```python
from build123d import *

# Parameters (mm, degrees)
BOSS_EXTRUDE1_DEPTH = 13.25
BOSS_EXTRUDE2_START = -2
BOSS_EXTRUDE2_DEPTH = 2
CHAMFER2_SIZE       = 2.5


with BuildPart() as part:
    # Sketch2 → Boss-Extrude1 (new, symmetric)
    with BuildSketch(Plane(origin=(0, 0, 0), x_dir=(1, 0, 0), z_dir=(0, 1, 0))):
        with BuildLine():
            Line((-52.61897195, 127.03343572), (-52.795575656, 127.459794782))
            Line((-52.795575656, 127.459794782), (-50.947816591, 128.225161647))
            Line((-50.947816591, 128.225161647), (-51.55131776, 129.682142355))
            Line((-51.55131776, 129.682142355), (-53.399076825, 128.91677549))
            Line((-53.399076825, 128.91677549), (-53.575680531, 129.343134552))
            ThreePointArc((-53.575680531, 129.343134552), (0, 140), (53.575680531, 129.343134552))
            Line((53.575680531, 129.343134552), (53.399076825, 128.91677549))
            Line((53.399076825, 128.91677549), (53.360808482, 128.824387537))
            Line((53.360808482, 128.824387537), (55.116179594, 128.097289015))
            Line((55.116179594, 128.097289015), (54.589215111, 126.825084214))
            Line((54.589215111, 126.825084214), (52.833843999, 127.552182735))
            Line((52.833843999, 127.552182735), (52.795575656, 127.459794782))
            Line((52.795575656, 127.459794782), (52.61897195, 127.03343572))
            ThreePointArc((52.61897195, 127.03343572), (0, 137.5), (-52.61897195, 127.03343572))
        make_face()
    extrude(amount=BOSS_EXTRUDE1_DEPTH, both=True)

    # Sketch3 → Boss-Extrude2 (add)
    with BuildSketch(Plane.XZ.offset(13.25).offset(BOSS_EXTRUDE2_START)):
        with BuildLine():
            ThreePointArc((53.575680531, -129.343134552), (0, -140), (-53.575680531, -129.343134552))
            Line((-53.575680531, -129.343134552), (-54.532389112, -131.652833383))
            ThreePointArc((-54.532389112, -131.652833383), (0, -142.5), (54.532389112, -131.652833383))
            Line((54.532389112, -131.652833383), (53.575680531, -129.343134552))
        make_face()
        with BuildLine():
            Line((-51.662263369, -124.723736889), (-52.61897195, -127.03343572))
            ThreePointArc((-52.61897195, -127.03343572), (0, -137.5), (52.61897195, -127.03343572))
            Line((52.61897195, -127.03343572), (51.662263369, -124.723736889))
            ThreePointArc((51.662263369, -124.723736889), (0, -135), (-51.662263369, -124.723736889))
        make_face()
    extrude(amount=BOSS_EXTRUDE2_DEPTH)

    # Chamfer2
    chamfer2_edges = [part.edges().sort_by_distance(p)[0] for p in [
        (0, -11.25, -137.5),
        (0, -11.25, -140),
    ]]
    chamfer(chamfer2_edges, length=CHAMFER2_SIZE - 0.0001)  # a hair under: the kernel refuses the full size


solid = part.part
```
Geometry: final body of the model. Coordinates: model frame, mm. A direction names the side the tool comes from. Round coordinates to 2 decimals unless told otherwise and drop trailing zeros. Write each loop counter-clockwise with the first axis right and the second up, starting at its lowest first coordinate (ties: lowest second). Pieces come first, ordered by that corner, then holes.
Item 1: Section query A-A (y = -3). Return loops of the section in (x, z).
Item 2: Set-up query: faces 1 (the face through (-52.462, 0.185, -129.305)), 2 (the face through (0.756, 2.404, -137.498)), 3 (the face through (-0.783, -12.236, -142.498)), 4 (the face through (0.7, -12.2, -135)), 5 (the face through (-51.88, 0.19, -127.84)). Return all of +Z, -Z, +X, -X, +Y, -Y with unobstructed straight access to the full face (end or side cutting, diameter ignored); none if empty.
Item 3: Mould query, pull axis X, two halves, no side actions, for faces 6 (the face through (-0.77, 2.404, -139.998)), 7 (the face through (54.226, 0.185, -128.466)), 8 (the face through (53.724, 0.185, -127.184)). Classes: +X half, -X half, draft (parallel to the pull), parting line (faces both ways), or undercut.
Item 4: Pin query (flat end, axial travel): P1, Ø1, axis at x = 38.5, y = -7.5, coming from the -Z side; P2, Ø5, axis at x = -25.5, y = 0.5, coming from the +Z side; P3, Ø8, axis at x = -21.5, z = -127.5, coming from the +Y side; P4, Ø8, axis at x = 20, y = -5, coming from the +Z side. Return the tip coordinate at first contact, or that it passes through.
Item 5: Material intervals for L1, parallel to X at y = 11, z = -128; L2, parallel to Z at x = 0.5, y = 11.5; L3, parallel to Z at x = 1.5, y = -11.5, sorted ascending.
Completed:
1. outline: (-53.58, -129.34) arc R140 ccw to (53.58, -129.34) - (53.36, -128.82) - (55.12, -128.1) - (54.59, -126.83) - (52.83, -127.55) - (52.62, -127.03) arc R137.5 cw to (-52.62, -127.03) - (-52.8, -127.46) - (-50.95, -128.23) - (-51.55, -129.68) - (-53.4, -128.92) - close
2. face 1: +Y, -Y
2. face 2: +Z, +Y
2. face 3: -Z, +Y, -Y
2. face 4: +Z, +Y, -Y
2. face 5: -X, +Y, -Y
3. face 6: parting line
3. face 7: +X half
3. face 8: undercut
4. P1: stops at z = -134.74
4. P2: stops at z = -134.62
4. P3: passes through
4. P4: stops at z = -135.39
5. L1: x = -51.49 to -50.22, 50.22 to 55.08
5. L2: z = -140 to -137.5
5. L3: z = -142.49 to -134.99
